```python
from build123d import *

# Parameters (mm, degrees)
SKETCH_1_W                  = 15
SKETCH_1_H                  = 15
SKETCH_1_W_2                = 12
SKETCH_1_H_2                = 12
EXTRUDE_1_DEPTH             = 568
SKETCH_5_R                  = 2.25
SKETCH_5_R_2                = 2.7
CUT_EXTRUDE_4_DEPTH         = 20
SKETCH_9_R                  = 2.7
CUT_EXTRUDE_6_DEPTH         = 40
SKETCH_10_R                 = 5
CUT_EXTRUDE_7_DEPTH         = 5
SKETCH_13_R                 = 2.25
CUT_EXTRUDE_10_DEPTH        = 40
SKETCH_14_R                 = 5
CUT_EXTRUDE_11_DEPTH        = 5
HOLE_WIZARD_10_0_10_1_D     = 10
HOLE_WIZARD_10_0_10_1_DEPTH = 1.5


with BuildPart() as part:
    # ｽｹｯﾁ1 → ﾎﾞｽ - 押し出し1 (new body)
    with BuildSketch(Plane.XY):
        Rectangle(SKETCH_1_W, SKETCH_1_H)
        Rectangle(SKETCH_1_W_2, SKETCH_1_H_2, mode=Mode.SUBTRACT)
    extrude(amount=EXTRUDE_1_DEPTH)

    # ｽｹｯﾁ5 → ｶｯﾄ - 押し出し4 (cut)
    with BuildSketch(Plane(origin=(0, -7.5, 0), x_dir=(-1, 0, 0), z_dir=(0, -1, 0))):
        with Locations((0, -22.5)):
            Circle(SKETCH_5_R)
        with Locations((0, -7.5)):
            Circle(SKETCH_5_R)
        with Locations((0, -560.5)):
            Circle(SKETCH_5_R)
        with Locations((0, -545.5)):
            Circle(SKETCH_5_R)
        with Locations((0, -42.5)):
            Circle(SKETCH_5_R_2)
        with Locations((0, -224)):
            Circle(SKETCH_5_R_2)
        with Locations((0, -344)):
            Circle(SKETCH_5_R_2)
        with Locations((0, -525.5)):
            Circle(SKETCH_5_R_2)
    extrude(amount=-CUT_EXTRUDE_4_DEPTH, mode=Mode.SUBTRACT)

    # ｽｹｯﾁ9 → ｶｯﾄ - 押し出し6 (cut)
    with BuildSketch(Plane(origin=(7.5, 0, 0), x_dir=(0, 0, -1), z_dir=(1, 0, 0))):
        with Locations((-494, 0)):
            Circle(SKETCH_9_R)
        with Locations((-399, 0)):
            Circle(SKETCH_9_R)
        with Locations((-202, 0)):
            Circle(SKETCH_9_R)
        with Locations((-157, 0)):
            Circle(SKETCH_9_R)
    extrude(amount=-CUT_EXTRUDE_6_DEPTH, mode=Mode.SUBTRACT)

    # ｽｹｯﾁ10 → ｶｯﾄ - 押し出し7 (cut)
    with BuildSketch(Plane.ZY.offset(7.5)):
        with Locations((157, 0)):
            Circle(SKETCH_10_R)
        with Locations((202, 0)):
            Circle(SKETCH_10_R)
        with Locations((399, 0)):
            Circle(SKETCH_10_R)
        with Locations((494, 0)):
            Circle(SKETCH_10_R)
    extrude(amount=-CUT_EXTRUDE_7_DEPTH, mode=Mode.SUBTRACT)

    # ｽｹｯﾁ13 → ｶｯﾄ - 押し出し10 (cut)
    with BuildSketch(Plane(origin=(7.5, 0, 0), x_dir=(0, 0, -1), z_dir=(1, 0, 0))):
        with Locations((-319, 0)):
            Circle(SKETCH_13_R)
        with Locations((-249, 0)):
            Circle(SKETCH_13_R)
    extrude(amount=-CUT_EXTRUDE_10_DEPTH, mode=Mode.SUBTRACT)

    # ｽｹｯﾁ14 → ｶｯﾄ - 押し出し11 (cut)
    with BuildSketch(Plane(origin=(7.5, 0, 0), x_dir=(0, 0, -1), z_dir=(1, 0, 0))):
        with Locations((-319, 0)):
            Circle(SKETCH_14_R)
        with Locations((-249, 0)):
            Circle(SKETCH_14_R)
    extrude(amount=-CUT_EXTRUDE_11_DEPTH, mode=Mode.SUBTRACT)

    # Ø10.0 (10) 直径の穴1
    with Locations(Plane(origin=(0, 7.5, 0), x_dir=(1, 0, 0), z_dir=(0, 1, 0))):
        with Locations((0, -42.5), (0, -224), (0, -344), (0, -525.5)):
            Hole(HOLE_WIZARD_10_0_10_1_D / 2, depth=HOLE_WIZARD_10_0_10_1_DEPTH)


solid = part.part
```
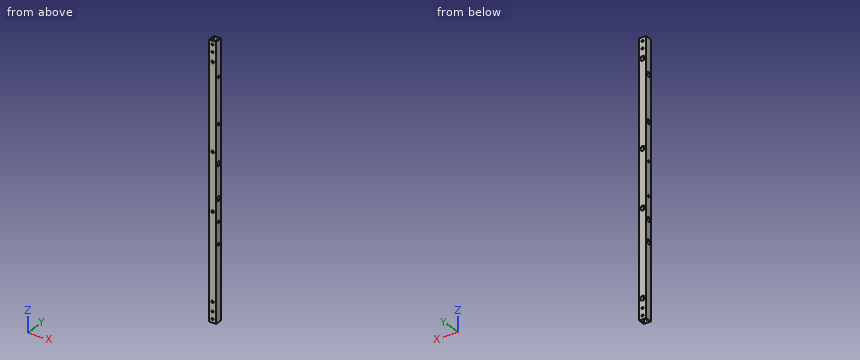
Here's how the part is built. I have some questions about the finished solid (model axes, mm). Coordinates: 2 decimals unless noted, no trailing zeros. Order: outer loops, then holes, each group sorted by start corner. A loop starts at its lowest first (then second) coordinate and runs counter-clockwise, first axis right, second up. Notation, with made-up numbers: M 38,-33.5 L 84,-33.5 A33 cw 84,-1.5 Z; hole C -24,60 d3. An arc over 180 degrees is marked long. Answer as a JSON object with one key per item and string values. Group by question number.
(1) Suppose I cut it at B-B, the plane x = 0. State how many separate pieces and enclosed holes the cut face has, then the cut area to 3 significant figures.
(2) Suppose I cut it at A-A, the plane z = 429. Please give me the cut outline in (x, y), then the cut area to 3 significant figures.
(3) I need wall thicknesses on probe 1 along X at (y, z) = (0.25, 525.5); probe 2 along Y at (x, z) = (6.45, 249). Which ranges of each line are inside material? Lowest first, please.
(4) For pin 1 (7 mm diameter, centred on x = 0, z = 224, fed in from +Y); pin 2 (5 mm diameter, centred on y = 0, z = 249, fed in from -X); pin 3 (3 mm diameter, centred on y = 1, z = 246, fed in from +X), each with a flat end and sliding along its axis, tell me the tip position at first contact or that it passes through.
Values found:
{
 "1": {"separate pieces": "18", "enclosed holes": "0", "area": "1,560 mm^2"},
 "2": {"outline": "M -7.5,-7.5 L 7.5,-7.5 L 7.5,7.5 L -7.5,7.5 Z; hole M -6,-6 L 6,-6 L 6,6 L -6,6 Z", "area": "81.0 mm^2"},
 "3": {"probe 1": "x = -7.5 to -6, 6 to 7.5", "probe 2": "y = -7.5 to -5, 5 to 7.5"},
 "4": {"pin 1": "stops at y = -6", "pin 2": "stops at x = -7.5", "pin 3": "stops at x = -6"}
}
